```python
from build123d import *

# Parameters (mm, degrees)
CYLINDER002_R     = 1.8
CYLINDER002_DEPTH = 50
ARRAY002_X_COUNT  = 2
ARRAY002_X_PITCH  = 27
ARRAY002_Y_COUNT  = 2
ARRAY002_Y_PITCH  = 15
BOX003_W          = 33
BOX003_H          = 21
BOX003_DEPTH      = 10


with BuildPart() as array002:
    # Cylinder002 → Cylinder002 (new body)
    with BuildSketch(Plane(origin=(3, 3, -10), x_dir=(1, 0, 0), z_dir=(0, 0, 1))):
        Circle(CYLINDER002_R)
    extrude(amount=CYLINDER002_DEPTH)

    # Array002 X: Array002 ×2


with BuildPart() as array002_1:
    add(array002.part)
    with Locations(*[(i * ARRAY002_X_PITCH, 0, 0) for i in range(1, ARRAY002_X_COUNT)]):
        add(array002.part)

    # Array002 Y: Array002 ×2


with BuildPart() as array002_2:
    add(array002_1.part)
    with Locations(*[(0, i * ARRAY002_Y_PITCH, 0) for i in range(1, ARRAY002_Y_COUNT)]):
        add(array002_1.part)


with BuildPart() as cut002:
    # Box003 → Box003 (new body)
    with BuildSketch(Plane.XY):
        with Locations((16.5, 10.5)):
            Rectangle(BOX003_W, BOX003_H)
    extrude(amount=BOX003_DEPTH)

    # Cut002: cut Array002
    add(array002_2.part, mode=Mode.SUBTRACT)


solid = cut002.part
```
Geometry check sheet. Reference: the model listing, model coordinates, mm. Coordinates: 2 decimals unless noted, no trailing zeros. Order: outer loops, then holes, each group sorted by start corner. A loop starts at its lowest first (then second) coordinate and runs counter-clockwise, first axis right, second up.
Q1. Sectioned sample at C-C on z = 7.5. Record the cut outline in (x, y), and give its area (3 significant figures).
Reply:
outline: (0, 0) - (33, 0) - (33, 21) - (0, 21) - close; hole circle Ø3.6 at (3, 3); hole circle Ø3.6 at (3, 18); hole circle Ø3.6 at (30, 3); hole circle Ø3.6 at (30, 18)
area: 652 mm2
Q2. Draft check along X on faces 1 (the face through (0, 10, 5)), 2 (the face through (2.766, 19.785, 4.93)), 3 (the face through (33, 10, 5)), 4 (the face through (16, 0, 5)). Enter one of: released by +X, released by -X, zero draft, split by the parting line, or undercut.
Reply:
face 1: released by -X
face 2: undercut
face 3: released by +X
face 4: zero draft
Q3. Thickness scan on probe 1 along Y at (x, z) = (30, 7.75); probe 2 along X at (y, z) = (18, 5.25); probe 3 along X at (y, z) = (18.5, 5.25). Record the ranges inside material, lowest first.
Reply:
probe 1: y = 0 to 1.2, 4.8 to 16.2, 19.8 to 21
probe 2: x = 0 to 1.2, 4.8 to 28.2, 31.8 to 33
probe 3: x = 0 to 1.27, 4.73 to 28.27, 31.73 to 33
Q4. Sectioned sample at A-A on y = 18. Record the cut outline in (x, z).
Reply:
outline: (0, 0) - (1.2, 0) - (1.2, 10) - (0, 10) - close; (4.8, 0) - (28.2, 0) - (28.2, 10) - (4.8, 10) - close; (31.8, 0) - (33, 0) - (33, 10) - (31.8, 10) - close
Q5. Sectioned sample at B-B on x = 3. Record the cut outline in (y, z), and give its area (3 significant figures).
Reply:
outline: (0, 0) - (1.2, 0) - (1.2, 10) - (0, 10) - close; (4.8, 0) - (16.2, 0) - (16.2, 10) - (4.8, 10) - close; (19.8, 0) - (21, 0) - (21, 10) - (19.8, 10) - close
area: 138 mm2
